Autodesk Inventor part; units mm, degrees
ref_plane "YZ Plane" through (0, 0, 0) normal (1, 0, 0) x (0, 1, 0)
ref_plane "XZ Plane" through (0, 0, 0) normal (0, 1, 0) x (-1, 0, 0)
ref_plane "XY Plane" through (0, 0, 0) normal (0, 0, 1) x (1, 0, 0)
sketch "Boceto1" plane through (0, 0, 0) normal (0, 1, 0) x (-1, 0, 0)
  line L0 (50, 10) -> (-50, 10)
  line L1 (-50, 10) -> (-50, -10)
  line L2 (-50, -10) -> (50, -10)
  line L3 (50, -10) -> (50, 10)
  line L4 (50, 10) -> (-50, -10) construction
  line L5 (-50, 10) -> (50, -10) construction
  line L6 (-50, -10) -> (-20, -10)
  line L7 (-20, -10) -> (0, 0)
  line L8 (0, 0) -> (50, 0)
  line L9 (0, 0) -> (0, 10)
  dimension "d0" = 100
  dimension "d1" = 20
  dimension "d2" = 30
extrude "Extrusión1" add sketch "Boceto1" along normal blind 5.5 contours L3 L8 L9 L0
extrude "Extrusión2" add sketch "Boceto1" along normal blind 5.5 contours L9 L7 L2 L1 L0
sketch "Boceto2" plane through (0, 5.5, 0) normal (0, 1, 0) x (1, 0, 0)
  line L0 (-50, 0) -> (-50, -10)
  line L1 (-50, -10) -> (-45, -10)
  line L2 (-50, -10) -> (50, -10)
  line L3 (-45, -10) -> (-45, 0)
  line L4 (0, 0) -> (-50, 0)
  arc A0 (-45, 0) -> (-45, -10) centre (-45, -5) ccw
  line L5 (-50, -5) -> (-25, -5)
  line L6 (-25, -5) -> (-25, 25)
  line L7 (-25, 25) -> (-15, 25)
  line L8 (-15, 25) -> (-15, -5)
  line L9 (-15, -5) -> (-25, -5)
  line L10 (-20, 25) -> (-20, 5)
  line L11 (-22.5, 7.5) -> (-17.5, 7.5)
  line L12 (-17.5, 7.5) -> (-17.5, 22.5)
  line L13 (-17.5, 22.5) -> (-22.5, 22.5)
  line L14 (-22.5, 22.5) -> (-22.5, 7.5)
  line L15 (-22.5, 7.5) -> (-17.5, 22.5) construction
  line L16 (-17.5, 7.5) -> (-22.5, 22.5) construction
  line L17 (-22.5, 22.5) -> (-22.5, 21.5)
  line L18 (-22.5, 21.5) -> (-17.5, 21.5)
  line L19 (-22.5, 15) -> (-17.5, 15)
  arc A1 (-17.5, 21.5) -> (-22.5, 21.5) centre (-20, 18.875) ccw
  arc A2 (-22.5, 8.5) -> (-17.5, 8.5) centre (-20, 11.125) ccw
  line L20 (-25, -5) -> (-20, -5)
  line L21 (-20, -5) -> (-20, -10)
  line L22 (-20, -10) -> (-25, -10)
  line L23 (-25, -10) -> (-25, -5)
  point P0 (0, -10)
  point P1 (-20, 15)
  point P2 (-50, -5)
  point P3 (-25, 0)
  point P4 (-15, 0)
  point P5 (-20, 22.5)
  point P6 (-20, 7.5)
  point P7 (-22.5, 8.5)
  point P8 (-17.5, 8.5)
  point P9 (-20, -5)
  dimension "d7" = 5
  dimension "d8" = 25
  dimension "d9" = 30
  dimension "d10" = 10
  dimension "d11" = 20
  dimension "d12" = 5
  dimension "d13" = 15
  dimension "d14" = 1
extrude "Extrusión3" cut sketch "Boceto2" against normal blind 5.5 contours L4 A0 L0 | A0 L1 L0
extrude "Extrusión4" add sketch "Boceto2" against normal blind 5.5 contours L6 L7 L8 L4 | L4 L8 L9 L6
extrude "Extrusión5" add sketch "Boceto2" against normal blind 5.5 contours A1 L14 L13 | L13 L12 A1 | A2 L12 L11 | L11 L14 A2
sketch "Boceto3" plane through (0, 5.5, 0) normal (0, 1, 0) x (1, 0, 0)
  arc A0 (-45, 0) -> (-45, -10) centre (-45, -5) ccw
  line L0 (-45, -5) -> (-43, -5)
  circle A1 centre (-43, -5) radius 3
  point P0 (0, 0)
  dimension "d21" = 2
  dimension "d22" = 6
extrude "Extrusión6" cut sketch "Boceto3" against normal blind 5.5
sketch "Boceto4" plane through (0, 5.5, 0) normal (0, 1, 0) x (1, 0, 0)
  line L0 (0, 0) -> (50, 0)
  line L1 (50, -10) -> (50, 10)
  line L2 (50, 10) -> (20, 10)
  line L3 (20, 10) -> (20, 0)
  line L4 (50, 0) -> (20, 0)
  circle A0 centre (35, 0) radius 25
  dimension "d27" = 50
extrude "Extrusión7" add sketch "Boceto4" against normal blind 5.5
sketch "Boceto5" plane through (0, 5.5, 0) normal (0, 1, 0) x (1, 0, 0)
  line L0 (-22.5, 8.5) -> (-22.5, 21.5)
  arc A0 (-22.5, 8.5) -> (-17.5, 8.5) centre (-20, 11.125) ccw
  line L1 (-17.5, 21.5) -> (-17.5, 8.5)
  circle A1 centre (-43, -5) radius 3
  line L2 (-43, -5) -> (-20, -5)
  line L3 (-20, -5) -> (-20, 11.125)
  line L4 (-20, 11.125) -> (-43, -5)
  line L5 (-22.5, 13.75) -> (-17.5, 13.75)
  point P0 (0, 0)
properties part number "PINZA_D"
The model under review builds one solid part; all positions refer to its coordinate system, in mm. A direction names the side the tool comes from. Coordinates: 2 decimals unless noted, no trailing zeros. Loops run counter-clockwise (first coordinate to the right, second up) from the corner with the lowest first, then second, coordinate; pieces in that order, holes last. Notation, with made-up numbers: (-7, 54.5) -> (40, 54.5) arc R36 ccw to (40, 89.5) -> close; hole circle Ø5 at (10.25, 61). An arc over 180 degrees is marked (long way). Use a Markdown table: item, result. Add a question column.
1. Add section C-C on z = 5. Write out the cut boundary in (x, y).
2. Add section A-A on x = -43. Write out the cut boundary in (y, z).
3. Machinability: for faces 5 (the face through (-20, 2.8, -22.5)), 6 (the face through (-35, 3, 0)), 7 (the face through (-15, 3, -13)), 8 (the face through (-17, 3, 10)), which of the approach directions +Z, -Z, +X, -X, +Y, -Y give a long, thin tool a straight path to every point of the face, cutting with its end or side? Answer none if there is none.
4. Add section D-D on z = -12. Write out the cut boundary in (x, y), plus the area to 3 significant figures.
5. Add section B-B on y = 4. Write out the cut boundary in (x, z) (3 decimals).
6. To check wall thickness, follow line 1 (Z direction, x = -43, y = 3.15); line 2 (X direction, y = 2.6, z = -14); line 3 (X direction, y = 0.25, z = -1). State the ranges of each line that lie inside material, in increasing order.
7. Clearance check with flat-ended pins moving along their axes: pin 1 Ø1 at (x, y) = (3, 3) entering from +Z; pin 2 Ø1 at (y, z) = (4, -1) entering from -X; pin 3 Ø2 at (x, y) = (19, 3) entering from -Z. State where each tip first meets the part, or that it passes through.
8. Draft analysis for pull direction Z (two halves, no side actions). For faces 1 (the face through (-17.5, 3, -15)), 2 (the face through (-20, 3, -25)), 3 (the face through (-50, 3, 5)), 4 (the face through (-22.5, 3, -15)), state which applies: pulls with the +Z half, pulls with the -Z half, needs draft (parallel to the pull), parting line crosses it, or undercut.
Returned:
| question | item | result |
|---|---|---|
| 1 | outline | (-50, 0) -> (-46, 0) -> (-46, 5.5) -> (-50, 5.5) -> close; (-40, 0) -> (59.49, 0) -> (59.49, 5.5) -> (-40, 5.5) -> close |
| 2 | outline | (0, 0) -> (5.5, 0) -> (5.5, 2) -> (0, 2) -> close; (0, 8) -> (5.5, 8) -> (5.5, 10) -> (0, 10) -> close |
| 3 | face 5 | +Y, -Y |
| 3 | face 6 | -Z, -X, +Y, -Y |
| 3 | face 7 | -Z, +Y, -Y |
| 3 | face 8 | +Z, -X, +Y, -Y |
| 4 | outline | (-25, 0) -> (-22.5, 0) -> (-22.5, 5.5) -> (-25, 5.5) -> close; (-17.5, 0) -> (-15, 0) -> (-15, 5.5) -> (-17.5, 5.5) -> close; (13.07, 0) -> (56.93, 0) -> (56.93, 5.5) -> (13.07, 5.5) -> close |
| 4 | area | 269 mm² |
| 5 | outline | (-45, 0) -> (-25, 0) -> (-25, -25) -> (-15, -25) -> (-15, 0) -> (0, 0) -> (10.564, -5.282) arc R25 ccw (long way) to (12.087, 10) -> (-45, 10) arc R5 ccw to start; hole circle Ø6 at (-43, 5); hole (-22.5, -21.5) arc R3.625 ccw to (-17.5, -21.5) -> (-17.5, -8.5) arc R3.625 ccw to (-22.5, -8.5) -> close |
| 6 | line 1 | z = 0 to 2, 8 to 10 |
| 6 | line 2 | x = -25 to -22.5, -17.5 to -15, 14.29 to 55.71 |
| 6 | line 3 | x = -25 to -15, 2 to 59.98 |
| 7 | pin 1 | stops at z = 10 |
| 7 | pin 2 | stops at x = -25 |
| 7 | pin 3 | stops at z = -20 |
| 8 | face 1 | undercut |
| 8 | face 2 | pulls with the -Z half |
| 8 | face 3 | parting line crosses it |
| 8 | face 4 | undercut |
